Autodesk Inventor part; units mm, degrees
ref_plane "Work Plane1" through (0, 20.0786, 47.2421) normal (0, 0, -1) x (-1, 0, 0)
ref_plane "YZ Plane" through (0, 0, 0) normal (1, 0, 0) x (0, 1, 0)
ref_plane "XZ Plane" through (0, 0, 0) normal (0, 1, 0) x (-1, 0, 0)
sketch "Sketch1" plane through (0, 0, 0) normal (1, 0, 0) x (0, 1, 0)
  line L0 (95.25, 0) -> (18.1319, 49.069)
  line L1 (0, 0) -> (0, -18.6) construction
  line L2 (95.25, 0) -> (4.9839, 0)
  line L3 (4.9839, 0) -> (18.1319, 49.069)
  dimension "d24" = 18.6
  dimension "d25" = 15
  dimension "d26" = 50.8
  dimension "d27" = 95.25
extrude "Extrusion1" add sketch "Sketch1" along normal blind 38.1
fillet "Fillet1" radius 3.175 3 edges at (19.05, 95.25, 0) (19.05, 4.9839, 0) (19.05, 18.1319, 49.069)
ref_plane "Work Plane1" through (0, 20.0786, 47.2421) normal (0, 0, -1) x (-1, 0, 0)
sketch "Sketch2" plane through (0, 20.0786, 47.2421) normal (0, 0, -1) x (-1, 0, 0)
  line L0 (0, 65.9715) -> (0, 1.7044)
  line L1 (-38.1, -14.0238) -> (0, -14.0238)
  point P0 (0, -20.0786)
  point P1 (-6.35, 56.1214)
  point P2 (-6.35, 30.7214)
  point P3 (-31.75, 56.1214)
  point P4 (-31.75, 30.7214)
  dimension "d28" = 76.2
  dimension "d29" = 6.35
  dimension "d32" = 25.4
  dimension "d35" = 25.4
hole "Hole1" at (6.35, 76.2, 47.2421) at (31.75, 76.2, 47.2421) at (6.35, 50.8, 47.2421) at (31.75, 50.8, 47.2421) direction (0, 0, -1) diameter 3.4036 end through all counterbore diameter 6.2992 counterbore depth 44.45
properties part number "CC-bottomStand" material "ABS Plastic"
Verification items for the finished model (mm, model axes). A direction names the side the tool comes from. Coordinates: 2 decimals unless noted, no trailing zeros. Loops run counter-clockwise (first coordinate to the right, second up) from the corner with the lowest first, then second, coordinate; pieces in that order, holes last. Notation, with made-up numbers: (53.25, 3) -> (74.25, 3) arc R18 cw to (74.25, 8) -> close; hole circle Ø11 at (85, 62). An arc over 180 degrees is marked (long way). Answer in a Markdown table with one row per item. Add a question column.
1. Section check A-A, the plane x = 31.75. Enter the section's corners in (y, z) (3 decimals), then the cut area to 3 significant figures.
2. Section check D-D, the plane x = 18.5. Enter the section's corners in (y, z) (3 decimals), then the cut area to 3 significant figures.
3. Section check B-B, the plane y = 50.8. Enter the section's corners in (x, z).
4. Depth check by flat-ended pin: P1, Ø5, axis at x = 31, y = 49.5, coming from the +Z side; P2, Ø1.5, axis at x = 16, z = 12, coming from the -Y side; P3, Ø2, axis at x = 20, y = 67.5, coming from the +Z side. Enter the tip coordinate at first touch or a pass-through.
5. Access from +Z, -Z, +X, -X, +Y, -Y to the whole of each face (thin tool, end or side, straight path). Record for faces 4 (the face through (31.7, 52.5, 1.4)), 5 (the face through (33.1, 74.8, 2.792)).
6. Section check C-C, the plane z = 8. Enter the section's corners in (x, y), then the cut area to 3 significant figures.
7. Material ranges on probe 1 along X at (y, z) = (76.2, 0.6); probe 2 along X at (y, z) = (76, 1); probe 3 along Y at (x, z) = (31.75, 1.9), recorded low to high. Write a range as [from, to].
8. Draft check along X on faces 1 (the face through (19, 47, 0)), 2 (the face through (38.1, 37, 19)), 3 (the face through (32.96, 73.29, 7.12)). Enter one of: +X half, -X half, draft (parallel to the pull), parting line (faces both ways), or undercut.
Derived:
| question | item | result |
|---|---|---|
| 1 | outline | (6.055, 3.997) arc R3.175 ccw to (9.122, 0) -> (49.098, 0) -> (49.098, 2.792) -> (47.65, 2.792) -> (47.65, 30.287) -> (21.783, 46.746) arc R3.175 ccw to (17.012, 44.889) -> close; (52.502, 0) -> (74.498, 0) -> (74.498, 2.792) -> (73.05, 2.792) -> (73.05, 14.125) -> (53.95, 26.279) -> (53.95, 2.792) -> (52.502, 2.792) -> close; (77.902, 0) -> (84.346, 0) arc R3.175 ccw to (86.05, 5.854) -> (79.35, 10.117) -> (79.35, 2.792) -> (77.902, 2.792) -> close |
| 1 | area | 1,950 mm² |
| 2 | outline | (6.055, 3.997) arc R3.175 ccw to (9.122, 0) -> (84.346, 0) arc R3.175 ccw to (86.05, 5.854) -> (21.783, 46.746) arc R3.175 ccw to (17.012, 44.889) -> close |
| 2 | area | 2,180 mm² |
| 3 | outline | (0, 0) -> (4.65, 0) -> (4.65, 2.79) -> (3.2, 2.79) -> (3.2, 28.28) -> (0, 28.28) -> close; (8.05, 0) -> (30.05, 0) -> (30.05, 2.79) -> (28.6, 2.79) -> (28.6, 28.28) -> (9.5, 28.28) -> (9.5, 2.79) -> (8.05, 2.79) -> close; (33.45, 0) -> (38.1, 0) -> (38.1, 28.28) -> (34.9, 28.28) -> (34.9, 2.79) -> (33.45, 2.79) -> close |
| 4 | P1 | stops at z = 30.7 |
| 4 | P2 | stops at y = 8 |
| 4 | P3 | stops at z = 18.29 |
| 5 | face 4 | +Z, -Z |
| 5 | face 5 | +Z |
| 6 | outline | (0, 7.13) -> (38.1, 7.13) -> (38.1, 82.68) -> (0, 82.68) -> close; hole circle Ø6.3 at (6.35, 50.8); hole circle Ø6.3 at (6.35, 76.2); hole circle Ø6.3 at (31.75, 50.8); hole circle Ø6.3 at (31.75, 76.2) |
| 6 | area | 2,750 mm² |
| 7 | probe 1 | x = [0, 4.65], [8.05, 30.05], [33.45, 38.1] |
| 7 | probe 2 | x = [0, 4.66], [8.04, 30.06], [33.44, 38.1] |
| 7 | probe 3 | y = [6.21, 49.1], [52.5, 74.5], [77.9, 87.25] |
| 8 | face 1 | draft |
| 8 | face 2 | +X half |
| 8 | face 3 | undercut |
